```python
from build123d import *

# Parameters (mm, degrees)
SKETCH1_W                     = 40
SKETCH1_H                     = 10
BOSS_EXTRUDE1_DEPTH           = 7.5
CBORE_FOR_M3_SHCS1_AT_2_COUNT = 2
CBORE_FOR_M3_SHCS1_AT_2_PITCH = 30
SKETCH4_W                     = 55
SKETCH4_H                     = 9.5
BOSS_EXTRUDE2_DEPTH           = 40
BOSS_EXTRUDE3_DEPTH           = 40
CUT_EXTRUDE1_DEPTH            = 70.282032303
CUT_EXTRUDE2_DEPTH            = 70.282032303


# Read off the part's stored shape, not the designer's step: Ø5.1 (5.1) Diameter Hole1
with BuildPart() as part:
    # Sketch1 → Boss-Extrude1 (new body)
    with BuildSketch(Plane.XY):
        with Locations((20, -5)):
            Rectangle(SKETCH1_W, SKETCH1_H)
    extrude(amount=BOSS_EXTRUDE1_DEPTH)

    # Sketch3 → CBORE for M3 SHCS1 (revolve, cut)
    with BuildSketch(Plane(origin=(35, -5, 7.5), x_dir=(0, -1, 0), z_dir=(1, 0, 0))):
        Polygon((0, 0), (0, 7.5), (1.7, 7.5), (1.7, 3), (3.25, 3), (3.25, 0.025), (3.275, 0), align=None)
    cbore_for_m3_shcs1 = revolve(axis=Axis((35, -5, 13.85), (0, 0, -1)), mode=Mode.SUBTRACT)

    # CBORE for M3 SHCS1 at 2: CBORE for M3 SHCS1 ×2
    with Locations(*[(-i * CBORE_FOR_M3_SHCS1_AT_2_PITCH, 0, 0) for i in range(1, CBORE_FOR_M3_SHCS1_AT_2_COUNT)]):
        add(cbore_for_m3_shcs1, mode=Mode.SUBTRACT)

    # Sketch4 → Boss-Extrude2 (add)
    with BuildSketch(Plane.XY):
        with Locations((12.5, 4.75)):
            Rectangle(SKETCH4_W, SKETCH4_H)
    extrude(amount=BOSS_EXTRUDE2_DEPTH)

    # Sketch5 → Boss-Extrude3 (add)
    with BuildSketch(Plane(origin=(0, 9.5, 0), x_dir=(1, 0, 0), z_dir=(0, 1, 0))):
        Polygon((-15, -5), (20, -40), (15, -40), (-15, -10), align=None)
    extrude(amount=BOSS_EXTRUDE3_DEPTH)

    # Sketch7 → Cut-Extrude1 (cut, through all)
    with BuildSketch(Plane(origin=(0, 9.5, 0), x_dir=(1, 0, 0), z_dir=(0, 1, 0))):
        Polygon((15, -40), (-15, -10), (-15, -40), align=None)
    extrude(amount=-CUT_EXTRUDE1_DEPTH, mode=Mode.SUBTRACT)

    # Ø5.1 (5.1) Diameter Hole1 outline → Ø5.1 (5.1) Diameter Hole1 (revolve, cut)
    with BuildSketch(Plane(origin=(23.106601718, 29.5, 23.106601718), x_dir=(0.7071067811865471, 0, 0.707106781186548), z_dir=(0, 1, 0))):
        Polygon((2.55, -17.65266953), (2.55, -14.142135624), (0, -14.142135624), (0, -17.67766953), (2.575, -17.67766953), align=None)
    revolve(axis=Axis((23.106601718, 29.5, 23.106601718), (0.707106781186548, 0, -0.7071067811865471)), mode=Mode.SUBTRACT)

    # 5.1 _5.1_ Diameter Hole1 2 outline → 5.1 _5.1_ Diameter Hole1 2 (revolve, cut)
    with BuildSketch(Plane(origin=(1.893398282, 29.5, 1.893398282), x_dir=(0.7071067811865471, 0, 0.707106781186548), z_dir=(0, 1, 0))):
        Polygon((2.55, -17.65266953), (2.55, -14.142135624), (0, -14.142135624), (0, -17.67766953), (2.575, -17.67766953), align=None)
    revolve(axis=Axis((1.893398282, 29.5, 1.893398282), (0.707106781186548, 0, -0.7071067811865471)), mode=Mode.SUBTRACT)

    # Sketch11 → Cut-Extrude2 (cut, through all)
    with BuildSketch(Plane(origin=(0, 9.5, 0), x_dir=(1, 0, 0), z_dir=(0, 1, 0))):
        Polygon((40, -20), (25, -40), (40, -40), align=None)
    extrude(amount=-CUT_EXTRUDE2_DEPTH, mode=Mode.SUBTRACT)


solid = part.part
```
Input: part model. Units: mm. Frame: model coordinates. A direction names the side the tool comes from. Coordinates: 2 decimals unless noted, no trailing zeros. Write each loop counter-clockwise with the first axis right and the second up, starting at its lowest first coordinate (ties: lowest second). Pieces come first, ordered by that corner, then holes. Notation, with made-up numbers: M 74.25,34.5 L 108.25,34.5 A29 cw 108.25,70.5 Z; hole C 72.5,51.5 d5. An arc over 180 degrees is marked long. Use one line per item in the form item = value.
Q1. Draft query along X for faces 1 (the face through (-8.36, 27.35, 14.09)), 2 (the face through (32.605, 4.816, 29.86)), 3 (the face through (19, 20, 40)). Return one class per face: released by +X, released by -X, zero draft, split by the parting line, or undercut.
Answer below:
face_1 = undercut
face_2 = released by +X
face_3 = zero draft
Q2. Section B-B (x = 5). Return loops of the section in (y, z) (3 decimals).
Answer below:
outline = M -10,0 L -6.7,0 L -6.7,4.5 L -8.25,4.5 L -8.25,7.475 L -8.275,7.5 L -10,7.5 Z; M -3.3,0 L 9.5,0 L 9.5,25 L 49.5,25 L 49.5,30 L 0,30 L 0,7.5 L -1.725,7.5 L -1.75,7.475 L -1.75,4.5 L -3.3,4.5 Z
Q3. Set-up query: faces 4 (the face through (2, 29, 22)), 5 (the face through (20, -5, 7.5)), 6 (the face through (4.02, -8.1, 6.01)), 7 (the face through (0, -5, 4)). Return all of +Z, -Z, +X, -X, +Y, -Y with unobstructed straight access to the full face (end or side cutting, diameter ignored); none if empty.
Answer below:
face_4 = -Z, +X, +Y
face_5 = +Z, +X, -X, -Y
face_6 = +Z
face_7 = +Z, -Z, -X, -Y
Q4. Section A-A (y = -5). Return loops of the section in (x, z) (3 decimals), plus the area to 3 significant figures.
Answer below:
outline = M 0,0 L 3.3,0 L 3.3,4.5 L 1.75,4.5 L 1.75,7.475 L 1.725,7.5 L 0,7.5 Z; M 6.7,0 L 33.3,0 L 33.3,4.5 L 31.75,4.5 L 31.75,7.475 L 31.725,7.5 L 8.275,7.5 L 8.25,7.475 L 8.25,4.5 L 6.7,4.5 Z; M 36.7,0 L 40,0 L 40,7.5 L 38.275,7.5 L 38.25,7.475 L 38.25,4.5 L 36.7,4.5 Z
area = 230 mm²
Q5. Material intervals for probe 1 along X at (y, z) = (-5, 5); probe 2 along X at (y, z) = (-5, 2); probe 3 along Y at (x, z) = (5, 6.05), sorted ascending. Write a range as from..to.
Answer below:
probe_1 = 0..1.75, 8.25..31.75, 38.25..40
probe_2 = 0..3.3, 6.7..33.3, 36.7..40
probe_3 = -10..-8.25, -1.75..9.5
Q6. Section C-C (x = 16.5). Return loops of the section in (y, z).
Answer below:
outline = M -10,0 L 9.5,0 L 9.5,36.5 L 49.5,36.5 L 49.5,40 L 0,40 L 0,7.5 L -10,7.5 Z
Q7. First-contact query: pin 1 (3 mm diameter, centred on x = 5.5, y = -6, fed in from +Z); pin 2 (4 mm diameter, centred on y = 19, z = 22, fed in from -X); pin 3 (12 mm diameter, centred on x = 21, z = 14.5, fed in from +Y); pin 4 (3 mm diameter, centred on x = 35, y = -5, fed in from -Z). Flat tips, straight axial feed; report the tip coordinate or a pass-through.
Answer below:
pin_1 = 4.5
pin_2 = -5
pin_3 = 9.5
pin_4 = through
Q8. Section D-D (y = 45). Return loops of the section in (x, z).
Answer below:
outline = M -15,5 L 20,40 L 15,40 L -15,10 Z
